Build history of the part. All positions in model axes, mm. Face numbers are marked on the shaded views. A direction names the side the tool comes from. Give positions to 0.01 mm unless a question says otherwise; leave off trailing zeros. Order: outer loops, then holes, each group sorted by start corner. A loop starts at its lowest first (then second) coordinate and runs counter-clockwise, first axis right, second up. Notation, with made-up numbers: (-9.75, -39) - (-4.75, -39) arc R27 ccw to (-4.75, -18) - close; hole circle Ø2 at (-3, 41). An arc over 180 degrees is marked (long way). Use a Markdown table: item, result.
from build123d import *

# Parameters (mm, degrees)
SKETCH1_R           = 18.9
BOSS_EXTRUDE1_DEPTH = 75
SKETCH2_R           = 1.5
CUT_EXTRUDE1_DEPTH  = 8
SKETCH3_R           = 2.5
BOSS_EXTRUDE2_DEPTH = 20
CUT_EXTRUDE4_START  = -20
SKETCH5_R           = 18.9
SKETCH5_R_2         = 17.9
CUT_EXTRUDE4_DEPTH  = 20
SKETCH6_R           = 18.9
SKETCH6_R_2         = 17.9
CUT_EXTRUDE5_DEPTH  = 20
SKETCH7_R           = 1.5
CUT_EXTRUDE6_DEPTH  = 99.688499837


with BuildPart() as part:
    # Sketch1 → Boss-Extrude1 (new body)
    with BuildSketch(Plane.XY):
        Circle(SKETCH1_R)
    extrude(amount=BOSS_EXTRUDE1_DEPTH)

    # Sketch2 → Cut-Extrude1 (cut)
    with BuildSketch(Plane.XY.offset(75)):
        with Locations((15.9, 0)):
            Circle(SKETCH2_R)
        with Locations((7.95, -13.76980392)):
            Circle(SKETCH2_R)
        with Locations((-7.95, -13.76980392)):
            Circle(SKETCH2_R)
        with Locations((-15.9, 0)):
            Circle(SKETCH2_R)
        with Locations((-7.95, 13.76980392)):
            Circle(SKETCH2_R)
        with Locations((7.95, 13.76980392)):
            Circle(SKETCH2_R)
    extrude(amount=-CUT_EXTRUDE1_DEPTH, mode=Mode.SUBTRACT)

    # Sketch3 → Boss-Extrude2 (add)
    with BuildSketch(Plane.XY.offset(75)):
        with Locations((0, -9.5)):
            Circle(SKETCH3_R)
    extrude(amount=BOSS_EXTRUDE2_DEPTH)

    # Sketch5 → Cut-Extrude4 (cut)
    with BuildSketch(Plane.XY.offset(75).offset(CUT_EXTRUDE4_START)):
        Circle(SKETCH5_R)
        Circle(SKETCH5_R_2, mode=Mode.SUBTRACT)
    extrude(amount=CUT_EXTRUDE4_DEPTH, mode=Mode.SUBTRACT)

    # Sketch6 → Cut-Extrude5 (cut)
    with BuildSketch(Plane(origin=(0, 0, 0), x_dir=(-1, 0, 0), z_dir=(0, 0, -1))):
        Circle(SKETCH6_R)
        with Locations(Location((0, 0, 0), (0, 0, 180))):
            Circle(SKETCH6_R_2, mode=Mode.SUBTRACT)
    extrude(amount=-CUT_EXTRUDE5_DEPTH, mode=Mode.SUBTRACT)

    # Sketch7 → Cut-Extrude6 (cut, through all)
    with BuildSketch(Plane(origin=(0, 0, 0), x_dir=(1, 0, 0), z_dir=(0, 1, 0))):
        with Locations(Location((0, -85, 0), (0, 0, 270))):
            Circle(SKETCH7_R)
    extrude(amount=-CUT_EXTRUDE6_DEPTH, mode=Mode.SUBTRACT)


solid = part.part
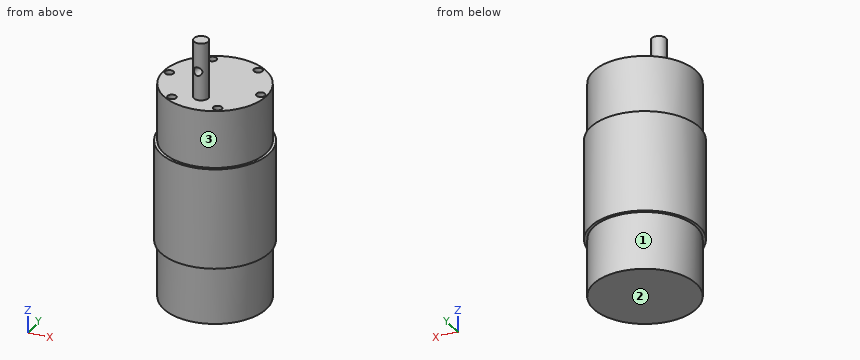
1) Slice it at C-C (y = -9.5). Write the cut outline in (x, z).
Computed:
| item | result |
|---|---|
| outline | (-16.34, 20) - (-15.17, 20) - (-15.17, 0) - (15.17, 0) - (15.17, 20) - (16.34, 20) - (16.34, 55) - (15.17, 55) - (15.17, 75) - (2.5, 75) - (2.5, 95) - (-2.5, 95) - (-2.5, 75) - (-15.17, 75) - (-15.17, 55) - (-16.34, 55) - close; hole circle Ø3 at (0, 85) |
2) Slice it at A-A (z = 85). Write the cut outline in (x, y), and give its area (3 significant figures).
Computed:
| item | result |
|---|---|
| outline | (-1.5, -11.5) - (-1.5, -7.5) arc R2.5 ccw to start; (1.5, -11.5) arc R2.5 ccw to (1.5, -7.5) - close |
| area | 5.59 mm² |
3) Slice it at D-D (x = 15.9). Write the cut outline in (y, z).
Computed:
| item | result |
|---|---|
| outline | (-10.22, 20) - (-8.22, 20) - (-8.22, 0) - (8.22, 0) - (8.22, 20) - (10.22, 20) - (10.22, 55) - (8.22, 55) - (8.22, 75) - (1.5, 75) - (1.5, 67) - (-1.5, 67) - (-1.5, 75) - (-8.22, 75) - (-8.22, 55) - (-10.22, 55) - close |
4) Slice it at B-B (y = 0). Write the cut outline in (x, z), and give its area (3 significant figures).
Computed:
| item | result |
|---|---|
| outline | (-18.9, 20) - (-17.9, 20) - (-17.9, 0) - (17.9, 0) - (17.9, 20) - (18.9, 20) - (18.9, 55) - (17.9, 55) - (17.9, 75) - (17.4, 75) - (17.4, 67) - (14.4, 67) - (14.4, 75) - (-14.4, 75) - (-14.4, 67) - (-17.4, 67) - (-17.4, 75) - (-17.9, 75) - (-17.9, 55) - (-18.9, 55) - close |
| area | 2,710 mm² |
5) Wall check: line 1 (Y direction, x = 7, z = 72); line 2 (Z direction, x = -8.5, y = -14.5); line 3 (Z direction, x = 0, y = -9.5). Give the ranges that are in metal, low to high. Write a range as from..to.
Computed:
| item | result |
|---|---|
| line 1 | y = -16.47..-14.93, -12.61..12.61, 14.93..16.47 |
| line 2 | z = 0..67 |
| line 3 | z = 0..83.5, 86.5..95 |
6) Pin check, flat tips, straight feed: P1, Ø0.9, axis at x = -8.5, y = 13.5, coming from the +Z side; P2, Ø5, axis at y = 4.5, z = 64.5, coming from the +X side; P3, Ø3.5, axis at x = -7.5, y = -13.5, coming from the +Z side. Stop position of each tip, or through.
Computed:
| item | result |
|---|---|
| P1 | stops at z = 67 |
| P2 | stops at x = 17.79 |
| P3 | stops at z = 75 |
7) Tool access for the marked faces 1, 2 and 3: list every direction of +Z, -Z, +X, -X, +Y, -Y with a clear straight run to the whole face (end or side of a thin tool).
Computed:
| item | result |
|---|---|
| face 1 | -Z |
| face 2 | -Z, +X, -X, +Y, -Y |
| face 3 | +Z |
